Here's how the part is built. I have some questions about the finished solid (model axes, mm). Round coordinates to 2 decimals unless told otherwise and drop trailing zeros. Order: outer loops, then holes, each group sorted by start corner. A loop starts at its lowest first (then second) coordinate and runs counter-clockwise, first axis right, second up. Notation, with made-up numbers: (-36.75, -19) - (-25.75, -19) arc R11 cw to (-25.75, -5) - close; hole circle Ø8 at (82.25, 49). An arc over 180 degrees is marked (long way). Answer as a JSON object with one key per item and string values.
```python
from build123d import *

# Parameters (mm, degrees)
SKETCH1_W           = 625
SKETCH1_H           = 590
BOSS_EXTRUDE1_DEPTH = 5
SKETCH2_W           = 395
SKETCH2_H           = 530
CUT_EXTRUDE1_DEPTH  = 23.4
CUT_EXTRUDE2_DEPTH  = 23.4


with BuildPart() as part:
    # Sketch1 → Boss-Extrude1 (new body)
    with BuildSketch(Plane(origin=(0, 0, 0), x_dir=(1, 0, 0), z_dir=(0, 1, 0))):
        Rectangle(SKETCH1_W, SKETCH1_H)
    extrude(amount=BOSS_EXTRUDE1_DEPTH)

    # Sketch2 → Cut-Extrude1 (cut)
    with BuildSketch(Plane(origin=(0, 5, 0), x_dir=(1, 0, 0), z_dir=(0, 1, 0))):
        with Locations((-85, 0)):
            Rectangle(SKETCH2_W, SKETCH2_H)
    extrude(amount=-CUT_EXTRUDE1_DEPTH, mode=Mode.SUBTRACT)

    # Sketch3 → Cut-Extrude2 (cut)
    with BuildSketch(Plane(origin=(0, 5, 0), x_dir=(1, 0, 0), z_dir=(0, 1, 0))):
        Polygon((112.5, 70), (112.5, 0), (112.5, -70), (212.5, -70), (212.5, 70), align=None)
    extrude(amount=-CUT_EXTRUDE2_DEPTH, mode=Mode.SUBTRACT)


solid = part.part
```
1. Imagine slicing it at B-B (z = -184). List the corners of the cut face in (x, y) for me, plus the area to 3 significant figures.
Responses:
{"outline": "(-312.5, 0) - (-282.5, 0) - (-282.5, 5) - (-312.5, 5) - close; (112.5, 0) - (312.5, 0) - (312.5, 5) - (112.5, 5) - close", "area": "1,150 mm2"}
2. If I drill on L1, parallel to X at y = 2.15, z = -52.5; L2, parallel to X at y = 2.15, z = -146.5; L3, parallel to Z at x = 123.5, y = 4.7, over which ranges is the centre line in solid material (lowest first)? Write a range as [from, to].
Responses:
{"L1": "[-312.5, -282.5], [212.5, 312.5]", "L2": "[-312.5, -282.5], [112.5, 312.5]", "L3": "[-295, -70], [70, 295]"}
3. Imagine slicing it at A-A (x = 163.5). List the corners of the cut face in (y, z) for me.
Responses:
{"outline": "(0, -295) - (5, -295) - (5, -70) - (0, -70) - close; (0, 70) - (5, 70) - (5, 295) - (0, 295) - close"}
4. Imagine slicing it at C-C (y = 3.15). List the corners of the cut face in (x, z) for me, plus the area to 3 significant figures.
Responses:
{"outline": "(-312.5, -295) - (312.5, -295) - (312.5, 295) - (-312.5, 295) - close; hole (-282.5, -265) - (112.5, -265) - (112.5, -70) - (212.5, -70) - (212.5, 70) - (112.5, 70) - (112.5, 265) - (-282.5, 265) - close", "area": "145,000 mm2"}
